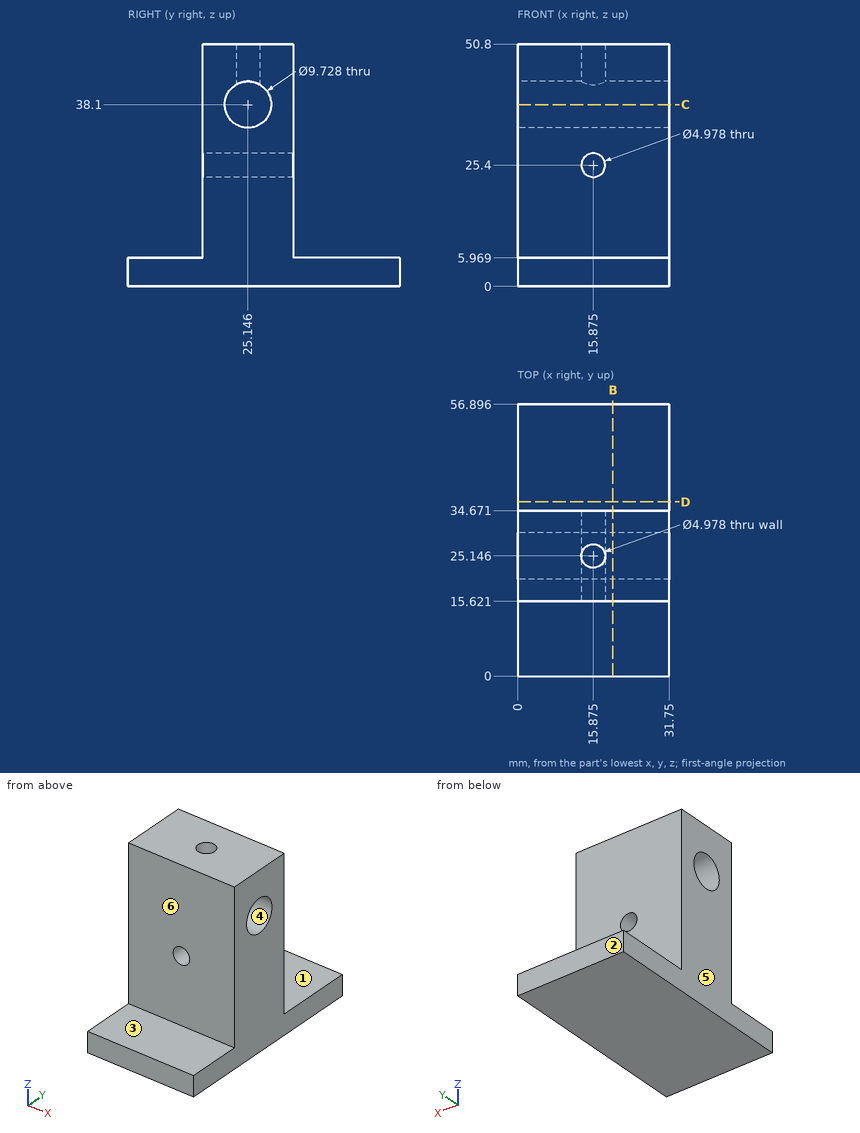
Print and shaded views of the part. All mm, measured from the part's lowest x, y and z. A direction names the side the tool comes from. Coordinates: 2 decimals unless noted, no trailing zeros. Order: outer loops, then holes, each group sorted by start corner. A loop starts at its lowest first (then second) coordinate and runs counter-clockwise, first axis right, second up. Notation, with made-up numbers: (7, 77) - (59, 77) arc R20 ccw to (59, 114) - close; hole circle Ø4 at (85.25, 51.5). An arc over 180 degrees is marked (long way). Put each result on its own line as item: value.
1. Tool access for the marked faces 1, 2 and 3: list every direction of +Z, -Z, +X, -X, +Y, -Y with a clear straight run to the whole face (end or side of a thin tool).
Answer sheet:
face 1: +Z, +X, -X, +Y
face 2: +Z, -Z, +X, -X, +Y
face 3: +Z, +X, -X, -Y
2. Drop flat-ended pins along their axis: P1, Ø4.5, axis at x = 11, y = 8, coming from the +Z side; P2, Ø6, axis at y = 47.5, z = 8, coming from the +X side; P3, Ø1.5, axis at x = 6.5, z = 23.5, coming from the +Y side; P4, Ø4, axis at x = 15.875, y = 25.146, coming from the +Z side. Give the stop position or say it passes through.
Answer sheet:
P1: stops at z = 5.97
P2: stops at x = 31.75
P3: stops at y = 34.67
P4: stops at z = 33.67
3. Saw through at D-D (y = 36.5). Write the cut outline in (x, z).
Answer sheet:
outline: (0, 0) - (31.75, 0) - (31.75, 5.97) - (0, 5.97) - close
4. Saw through at B-B (x = 20). Write the cut outline in (y, z).
Answer sheet:
outline: (0, 0) - (56.9, 0) - (56.9, 5.97) - (34.67, 5.97) - (34.67, 50.8) - (15.62, 50.8) - (15.62, 5.97) - (0, 5.97) - close; hole circle Ø9.73 at (25.15, 38.1)
5. Saw through at C-C (z = 38.1). Write the cut outline in (x, y).
Answer sheet:
outline: (0, 15.62) - (31.75, 15.62) - (31.75, 20.28) - (0, 20.28) - close; (0, 30.01) - (31.75, 30.01) - (31.75, 34.67) - (0, 34.67) - close
6. Probe line 1 along Z through (x, y) = (30.5, 37); line 2 along Y through (x, z) = (18, 32); line 3 along Z through (x, y) = (30.5, 22.5). List the from-to ranges inside material, lowest first. Write a range as [from, to].
Answer sheet:
line 1: z = [0, 5.97]
line 2: y = [15.62, 34.67]
line 3: z = [0, 34.02], [42.18, 50.8]
7. Pull direction Y, two halves, no side cores. Call the marked faces 4, 5 and 6: pulls with the +Y half, pulls with the -Y half, needs draft (parallel to the pull), parting line crosses it, or undercut.
Answer sheet:
face 4: undercut
face 5: needs draft
face 6: pulls with the -Y half
